from build123d import *

# Parameters (mm, degrees)
SKETCH1_R               = 62.5
BOSS_EXTRUDE3_DEPTH     = 223
CUT_EXTRUDE1_DEPTH      = 240.878094039
CUT_EXTRUDE1_DEPTH_BACK = 172
SKETCH3_W               = 51
SKETCH3_H               = 1
CUT_EXTRUDE2_DEPTH      = 174


with BuildPart() as part:
    # Sketch1 → Boss-Extrude3 (new body)
    with BuildSketch(Plane.XY):
        with Locations(Location((0, 0, 0), (0, 0, 180))):
            Circle(SKETCH1_R)
    extrude(amount=BOSS_EXTRUDE3_DEPTH)

    # Sketch2 → Cut-Extrude1 (cut, two sides: drawn at the far end of the back side and taken through both)
    with BuildSketch(Plane(origin=(0, 0, 0), x_dir=(-1, 0, 0), z_dir=(0, 0, -1)).offset(-CUT_EXTRUDE1_DEPTH_BACK)):
        Polygon((-360.670689192, 38.157568057), (-49.5, 38.157568057), (49.5, 38.157568057), (360.670689192, 38.157568057), (360.670689192, 660.498946441), (-360.670689192, 660.498946441), align=None)
    extrude(amount=CUT_EXTRUDE1_DEPTH + CUT_EXTRUDE1_DEPTH_BACK, mode=Mode.SUBTRACT)

    # Sketch3 → Cut-Extrude2 (cut)
    with BuildSketch(Plane(origin=(-62.5, 0, 0), x_dir=(0, 0, -1), z_dir=(1, 0, 0))):
        with Locations((-197.5, 62)):
            Rectangle(SKETCH3_W, SKETCH3_H)
    extrude(amount=CUT_EXTRUDE2_DEPTH, mode=Mode.SUBTRACT)


solid = part.part
Input: part model. Units: mm. Frame: model coordinates. A direction names the side the tool comes from. Coordinates: 2 decimals unless noted, no trailing zeros. Loops run counter-clockwise (first coordinate to the right, second up) from the corner with the lowest first, then second, coordinate; pieces in that order, holes last.
(1) First-contact query: pin 1 Ø11.5 at (x, y) = (-11.5, 51.5) entering from -Z; pin 2 Ø12 at (y, z) = (-43.5, 79) entering from +X; pin 3 Ø12 at (x, z) = (-36.5, 102.5) entering from -Y; pin 4 Ø12 at (x, y) = (47.5, 41.5) entering from -Z. Flat tips, straight axial feed; report the tip coordinate or a pass-through.
(2) Section B-B on y = -50. Return the cut outline in (x, z), then the cut area to 3 significant figures.
(3) Section A-A on x = 0. Return the cut outline in (y, z).
(4) Material intervals for probe 1 along Z at (x, y) = (-0.5, 49.5); probe 2 along Y at (x, z) = (1, 159.5); probe 3 along Y at (x, z) = (-42, 204), sorted ascending.
(5) Section D-D on x = -17. Return the cut outline in (y, z), then the cut area to 3 significant figures.
(6) Section C-C on z = 43.5. Return the cut outline in (x, y).
(7) Set-up query: faces 1 (the face through (1, -13, 0)), 2 (the face through (1, 38.158, 87)). Return all of +Z, -Z, +X, -X, +Y, -Y with unobstructed straight access to the full face (end or side cutting, diameter ignored); none if empty.
Data:
1. pin 1: stops at z = 172
1. pin 2: stops at x = 50
1. pin 3: stops at y = -54.55
1. pin 4: stops at z = 0
2. outline: (-37.5, 0) - (37.5, 0) - (37.5, 223) - (-37.5, 223) - close
2. area: 16,700 mm2
3. outline: (-62.5, 0) - (38.16, 0) - (38.16, 172) - (61.5, 172) - (61.5, 223) - (-62.5, 223) - close
4. probe 1: z = 172 to 223
4. probe 2: y = -62.49 to 38.16
4. probe 3: y = -46.28 to 46.28
5. outline: (-60.14, 0) - (38.16, 0) - (38.16, 172) - (60.14, 172) - (60.14, 223) - (-60.14, 223) - close
5. area: 23,000 mm2
6. outline: (-49.5, 38.16) arc R62.5 ccw (long way) to (49.5, 38.16) - close
7. face 1: -Z, +X, -X, +Y, -Y
7. face 2: -Z, +X, -X, +Y
